```python
from build123d import *

# Parameters (mm, degrees)
F0_W     = 12.7
F0_H     = 27.606282
F1_DEPTH = 25.4
F2_DEPTH = 15.24
F3_R     = 5.08
F4_DEPTH = 25.4


with BuildPart() as f1:
    # F0 (on Top) → F1 (new body)
    with BuildSketch(Plane.XY):
        with Locations((-251.110267, -68.915142)):
            Rectangle(F0_W, F0_H)
    extrude(amount=F1_DEPTH)

    # F0 (on Top) → F2 (join)
    with BuildSketch(Plane.XY):
        Polygon((-171.100267, 33.879176), (-298.100267, 33.879176), (-298.100267, -49.940824), (-260.000267, -49.940824), (-234.600267, -49.940824), (-171.100267, -49.940824), align=None)
        with Locations((-251.110267, -68.915142)):
            Rectangle(F0_W, F0_H)
        Polygon((-234.600267, -49.940824), (-260.000267, -49.940824), (-260.000267, -82.718283), (-257.460267, -82.718283), (-257.460267, -55.112001), (-244.760267, -55.112001), (-244.760267, -82.718283), (-234.600267, -82.718283), align=None)
    extrude(amount=-F2_DEPTH)

    # F3 (on face) → F4 (cut)
    with BuildSketch(Plane(origin=(-257.460267, 0, 0), x_dir=(0, -1, 0), z_dir=(-1, 0, 0))):
        with Locations((67.812001, 14.478)):
            Circle(F3_R)
    extrude(amount=-F4_DEPTH, mode=Mode.SUBTRACT)


solid = f1.part
```
Source: CAD feature listing. Evaluate the final solid. Frame: model axes, mm. A direction names the side the tool comes from. Coordinates: 2 decimals unless noted, no trailing zeros. Write each loop counter-clockwise with the first axis right and the second up, starting at its lowest first coordinate (ties: lowest second). Pieces come first, ordered by that corner, then holes. Notation, with made-up numbers: (41, 65) - (59, 65) arc R9 cw to (59, 76) - close; hole circle Ø8 at (69.25, 9). An arc over 180 degrees is marked (long way). Answer as a JSON object with one key per item and string values.
Q1. Section query C-C, the plane z = -6. Output: boundary loops of the cut face in (x, y).
Ans:
{"outline": "(-298.1, -49.94) - (-260, -49.94) - (-260, -82.72) - (-234.6, -82.72) - (-234.6, -49.94) - (-171.1, -49.94) - (-171.1, 33.88) - (-298.1, 33.88) - close"}
Q2. First-contact query: pin 1 Ø10 at (x, y) = (-212, -42) entering from +Z; pin 2 Ø11.5 at (y, z) = (-67.812, 14.478) entering from -X; pin 3 Ø12 at (y, z) = (-69, -7) entering from +X. Flat tips, straight axial feed; report the tip coordinate or a pass-through.
Ans:
{"pin 1": "stops at z = 0", "pin 2": "stops at x = -257.46", "pin 3": "stops at x = -234.6"}
Q3. Section query D-D, the plane y = -52. Output: boundary loops of the cut face in (x, z).
Ans:
{"outline": "(-260, -15.24) - (-234.6, -15.24) - (-234.6, 0) - (-260, 0) - close"}
Q4. Material intervals for line 1 (Z direction, x = -242, y = -42); line 2 (Y direction, x = -230, z = -1); line 3 (X direction, y = -58.5, z = 1), sorted ascending. Write a range as [from, to].
Ans:
{"line 1": "z = [-15.24, 0]", "line 2": "y = [-49.94, 33.88]", "line 3": "x = [-257.46, -244.76]"}
Q5. Section query B-B, the plane y = -69. Output: boundary loops of the cut face in (x, z), plus the area to 3 significant figures.
Ans:
{"outline": "(-260, -15.24) - (-234.6, -15.24) - (-234.6, 0) - (-244.76, 0) - (-244.76, 9.54) - (-257.46, 9.54) - (-257.46, 0) - (-260, 0) - close; (-257.46, 19.42) - (-244.76, 19.42) - (-244.76, 25.4) - (-257.46, 25.4) - close", "area": "584 mm2"}
Q6. Draft query along Z for faces 4 (the flat face through (-250, -82.718, 1)), 5 (the cylindrical face through (-251.2, -63.78, 11.39)), 6 (the flat face through (-235, -11, -15.24)). Return one class per face: released by +Z, released by -Z, zero draft, split by the parting line, or undercut.
Ans:
{"face 4": "zero draft", "face 5": "undercut", "face 6": "released by -Z"}
Q7. Section query A-A, the plane x = -248. Output: boundary loops of the cut face in (y, z), plus the area to 3 significant figures.
Ans:
{"outline": "(-82.72, -15.24) - (33.88, -15.24) - (33.88, 0) - (-55.11, 0) - (-55.11, 25.4) - (-82.72, 25.4) - close; hole circle Ø10.16 at (-67.81, 14.48)", "area": "2,400 mm2"}
Q8. Set-up query: faces 1 (the flat face through (-244.76, -72, 10)), 2 (the flat face through (-251, -55.112, 13)), 3 (the flat face through (-234.6, -67, -8)). Return all of +Z, -Z, +X, -X, +Y, -Y with unobstructed straight access to the full face (end or side cutting, diameter ignored); none if empty.
Ans:
{"face 1": "+Z, +X, +Y, -Y", "face 2": "+Z, +X, -X, +Y", "face 3": "+Z, -Z, +X, -Y"}
